For this review, use the dimensioned drawing (mm, ordinates from the lowest corner) and the shaded views. Give positions to 0.01 mm unless a question says otherwise; leave off trailing zeros. Write each loop counter-clockwise with the first axis right and the second up, starting at its lowest first coordinate (ties: lowest second). Pieces come first, ordered by that corner, then holes. Notation, with made-up numbers: M -33,-12.5 L 21,-12.5 A34 cw 21,26.5 Z; hole C 39,-37.75 d9. An arc over 180 degrees is marked long. Answer in a Markdown table with one row per item.
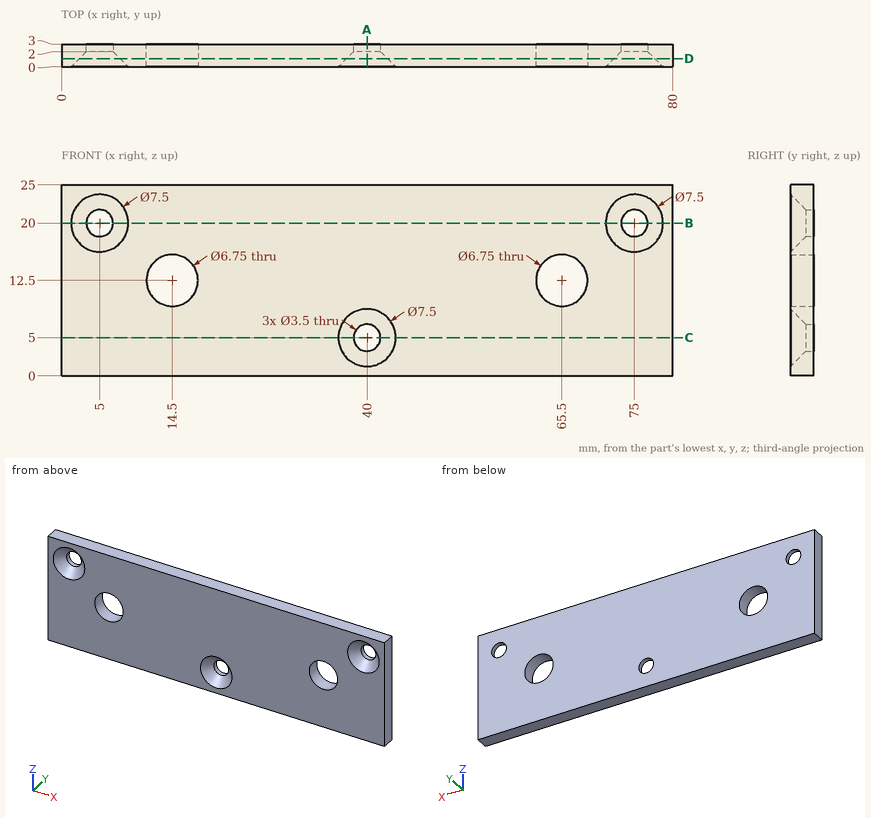
1) Add section B-B (z = 20). Write out the cut boundary in (x, y).
Geometry says:
| item | result |
|---|---|
| outline | M 0,0 L 1.25,0 L 3.25,2 L 3.25,3 L 0,3 Z; M 6.75,2 L 8.75,0 L 71.25,0 L 73.25,2 L 73.25,3 L 6.75,3 Z; M 76.75,2 L 78.75,0 L 80,0 L 80,3 L 76.75,3 Z |
2) Insertion check: P1, Ø6, axis at x = 65.5, z = 12.5, coming from the -Y side; P2, Ø4.5, axis at x = 75, z = 20, coming from the -Y side. Each pin has a flat end and moves straight along its axis. Give the tip position at first contact, or say it passes through.
Geometry says:
| item | result |
|---|---|
| P1 | through |
| P2 | y = 1.5 |
3) Add section D-D (y = 1.1). Write out the cut boundary in (x, z) (3 decimals).
Geometry says:
| item | result |
|---|---|
| outline | M 0,0 L 80,0 L 80,25 L 0,25 Z; hole C 5,20 d5.3; hole C 14.5,12.5 d6.75; hole C 40,5 d5.3; hole C 65.5,12.5 d6.75; hole C 75,20 d5.3 |
4) Add section C-C (z = 5). Write out the cut boundary in (x, y).
Geometry says:
| item | result |
|---|---|
| outline | M 0,0 L 36.25,0 L 38.25,2 L 38.25,3 L 0,3 Z; M 41.75,2 L 43.75,0 L 80,0 L 80,3 L 41.75,3 Z |
5) To check wall thickness, follow probe 1 along Z at (x, y) = (65.5, 0.6) (3 decimals); probe 2 along X at (y, z) = (1.05, 15.25); probe 3 along Z at (x, y) = (5, 2.7). State the ranges of each line that lie inside material, in increasing order. Write a range as [from, to].
Geometry says:
| item | result |
|---|---|
| probe 1 | [0, 9.125], [15.875, 25] |
| probe 2 | [0, 12.54], [16.46, 63.54], [67.46, 80] |
| probe 3 | [0, 18.25], [21.75, 25] |
6) Add section A-A (x = 40). Write out the cut boundary in (y, z), and give its area (3 significant figures).
Geometry says:
| item | result |
|---|---|
| outline | M 0,0 L 3,0 L 3,3.25 L 2,3.25 L 0,1.25 Z; M 0,8.75 L 2,6.75 L 3,6.75 L 3,25 L 0,25 Z |
| area | 60.5 mm^2 |
